```python
from build123d import *

# Parameters (mm, degrees)
SKETCH1_R           = 22
BOSS_EXTRUDE1_DEPTH = 4.5
BOSS_EXTRUDE2_START = 4.5
SKETCH2_R           = 11.25
BOSS_EXTRUDE2_DEPTH = 2
BOSS_EXTRUDE3_START = 4.5
SKETCH3_R           = 3.5
BOSS_EXTRUDE3_DEPTH = 2
BOSS_EXTRUDE4_START = 6.5
SKETCH4_R           = 4
BOSS_EXTRUDE4_DEPTH = 10
CUT_EXTRUDE1_START  = 16.5
SKETCH5_W           = 54.287880581
SKETCH5_H           = 2
CUT_EXTRUDE1_DEPTH  = 5
SKETCH6_R           = 13
CUT_EXTRUDE2_DEPTH  = 4


with BuildPart() as part:
    # Sketch1 → Boss-Extrude1 (new body)
    with BuildSketch(Plane.XY):
        Circle(SKETCH1_R)
    extrude(amount=BOSS_EXTRUDE1_DEPTH)

    # Sketch2 → Boss-Extrude2 (add)
    with BuildSketch(Plane.XY.offset(BOSS_EXTRUDE2_START)):
        Circle(SKETCH2_R)
    extrude(amount=BOSS_EXTRUDE2_DEPTH)

    # Sketch3 → Boss-Extrude3 (add)
    with BuildSketch(Plane.XY.offset(BOSS_EXTRUDE3_START)):
        with Locations((-4.210444621, 16.315472905)):
            Circle(SKETCH3_R)
    extrude(amount=BOSS_EXTRUDE3_DEPTH)

    # Sketch4 → Boss-Extrude4 (add)
    with BuildSketch(Plane.XY.offset(BOSS_EXTRUDE4_START)):
        Circle(SKETCH4_R)
    extrude(amount=BOSS_EXTRUDE4_DEPTH)

    # Sketch5 → Cut-Extrude1 (cut)
    with BuildSketch(Plane.XY.offset(CUT_EXTRUDE1_START)):
        with Locations((2.276588541, 0)):
            Rectangle(SKETCH5_W, SKETCH5_H)
    extrude(amount=-CUT_EXTRUDE1_DEPTH, mode=Mode.SUBTRACT)

    # Sketch6 → Cut-Extrude2 (cut)
    with BuildSketch(Plane.XY):
        Circle(SKETCH6_R)
    extrude(amount=CUT_EXTRUDE2_DEPTH, mode=Mode.SUBTRACT)


solid = part.part
```
Here's how the part is built. I have some questions about the finished solid (model axes, mm). A direction names the side the tool comes from. Give positions to 0.01 mm unless a question says otherwise; leave off trailing zeros. Loops run counter-clockwise (first coordinate to the right, second up) from the corner with the lowest first, then second, coordinate; pieces in that order, holes last. Notation, with made-up numbers: M 89.5,14.5 L 140.5,14.5 A23 ccw 140.5,36.5 Z; hole C -35,44.25 d2. An arc over 180 degrees is marked long. Use one line per item in the form item = value. Start each with the question number.
Q1. Thinking about a two-plate mould opening in X: for faces 1 (the cylindrical face through (-4.666, 19.786, 5.486)), 2 (the flat face through (0, 0, 4)), 3 (the flat face through (0, -1, 14)), which applies, +X half, -X half, draft (parallel to the pull), parting line (faces both ways), or undercut?
Q2. If we section it at B-B (x = 0): Write out the boundary of the cut face in (y, z).
Q3. Will these pins go through, and if not, where does the flat tip stop? pin 1 Ø3.5 at (x, y) = (-4.5, 15.5) entering from +Z; pin 2 Ø4 at (x, z) = (-2, 14.5) entering from +Y; pin 3 Ø2 at (x, y) = (-13, 12.5) entering from +Z; pin 4 Ø3 at (x, z) = (-16, 6.5) entering from -Y.
Q4. I need wall thicknesses on line 1 along Y through (x, z) = (0, 1.15); line 2 along Z through (x, y) = (-7.5, -9); line 3 along Z through (x, y) = (3.5, 17). Which ranges of each line are inside material? Lowest first, please.
Q5. Which directions (+Z, -Z, +X, -X, +Y, -Y) give clear straight access to the entire face, cutting with the end or side of a thin tool? Please do faces 4 (the flat face through (-4, 16, 6.5)), 5 (the flat face through (0, 0, 11.5)), 6 (the cylindrical face through (5.19, -9.98, 5.49)).
Q6. If we section it at C-C (z = 15.5): Write out the boundary of the cut face in (x, y).
Q7. If we section it at A-A (y = 0): Write out the boundary of the cut face in (x, z).
Q8. If we section it at D-D (z = 8.25): Write out the boundary of the cut face in (x, y).
Taken from the geometry:
q1.face_1 = parting line
q1.face_2 = undercut
q1.face_3 = draft
q2.outline = M -22,0 L -13,0 L -13,4 L 13,4 L 13,0 L 22,0 L 22,4.5 L 11.25,4.5 L 11.25,6.5 L 4,6.5 L 4,16.5 L 1,16.5 L 1,11.5 L -1,11.5 L -1,16.5 L -4,16.5 L -4,6.5 L -11.25,6.5 L -11.25,4.5 L -22,4.5 Z
q3.pin_1 = 6.5
q3.pin_2 = 4
q3.pin_3 = 4.5
q3.pin_4 = through
q4.line_1 = -22 to -13, 13 to 22
q4.line_2 = 4 to 4.5
q4.line_3 = 0 to 4.5
q5.face_4 = +Z, +X, -X, +Y
q5.face_5 = +Z, +X, -X
q5.face_6 = +Z
q6.outline = M -3.87,-1 A4 ccw 3.87,-1 Z; M -3.87,1 L 3.87,1 A4 ccw Z
q7.outline = M -22,0 L -13,0 L -13,4 L 13,4 L 13,0 L 22,0 L 22,4.5 L 11.25,4.5 L 11.25,6.5 L 4,6.5 L 4,11.5 L -4,11.5 L -4,6.5 L -11.25,6.5 L -11.25,4.5 L -22,4.5 Z
q8.outline = C 0,0 d8
